The model under review builds one solid part; all positions refer to its coordinate system, in mm. A direction names the side the tool comes from. Round coordinates to 2 decimals unless told otherwise and drop trailing zeros. Write each loop counter-clockwise with the first axis right and the second up, starting at its lowest first coordinate (ties: lowest second). Pieces come first, ordered by that corner, then holes. Notation, with made-up numbers: M -23.75,18.5 L -10.75,18.5 A7 ccw -10.75,23.5 Z; hole C -16,47.25 d11. An arc over 180 degrees is marked long. One line per item, written item: value. Start each with the question number.
1) For P1, Ø1.5, axis at y = 19.5, z = 4, coming from the +X side; P2, Ø3.5, axis at x = -0.5, y = 53, coming from the -Z side; P3, Ø5, axis at x = 0.5, y = -52.5, coming from the -Z side (3 decimals); P4, Ø0.7, axis at x = 0.5, z = -2.5, coming from the -Y side, all flat-tipped, find the tip position at first contact; note any pin that passes through.
2) Take a section at A-A, the plane y = 11. Write out the cut boundary in (x, z) (1 decimal), and give its area (3 significant figures).
3) Tool access review of faces 1 (the face through (-2, 55.562, 2)), 2 (the face through (-0.69, 45.65, -3.1)), 3 (the face through (0, 53, 2.245)), 4 (the face through (2.245, -53, 0)): name each direction out of +Z, -Z, +X, -X, +Y, -Y from which nothing blocks a thin tool from reaching the whole face with its end or side.
4) Take a section at B-B, the plane y = 57. Write out the cut boundary in (x, z).
5) Wall thickness on probe 1 along Y at (x, z) = (3, -3.25); probe 2 along Z at (x, y) = (-1.5, 52); probe 3 along X at (y, z) = (57.5, -1.5): over which ranges is each line inside the solid? List them lowest first.
from build123d import *

# Parameters (mm, degrees)
F0_R     = 3.175
F1_DEPTH = 50.8
F2_W     = 4.490128
F2_H     = 4.490128
F3_DEPTH = 4.7625
F4_R     = 2.245064
F5_DEPTH = 12.7
F6_R     = 4.7625
F7_DEPTH = 40.64


with BuildPart() as f1:
    # F0 (on Front) → F1 (new body)
    with BuildSketch(Plane.XZ):
        Circle(F0_R)
    extrude(amount=F1_DEPTH)

    # F2 (on face) → F3 (join)
    with BuildSketch(Plane.XZ.offset(50.8)):
        Rectangle(F2_W, F2_H)
    extrude(amount=F3_DEPTH)

    # F4 (on face) → F5 (join)
    with BuildSketch(Plane.XZ.offset(55.5625)):
        Circle(F4_R)
    extrude(amount=F5_DEPTH)

    # F6 (on face) → F7 (join)
    with BuildSketch(Plane(origin=(0, 0, 0), x_dir=(-1, 0, 0), z_dir=(0, 1, 0))):
        Circle(F6_R)
    extrude(amount=-F7_DEPTH)

    # F8: F1 across plane


with BuildPart() as f1_1:
    add(f1.part)
    add(f1.part.mirror(Plane.XZ))


solid = f1_1.part
Checked values:
1. P1: stops at x = 3.48
1. P2: stops at z = -2.25
1. P3: stops at z = -3.175
1. P4: stops at y = -68.26
2. outline: C 0,0 d9.5
2. area: 71.3 mm2
3. face 1: +Z, -X, +Y
3. face 2: +Y
3. face 3: +Z, +X, -X, +Y
3. face 4: +Z, -Z, +X, -Y
4. outline: C 0,0 d4.49
5. probe 1: y = -40.64 to 40.64
5. probe 2: z = -2.25 to 2.25
5. probe 3: x = -1.67 to 1.67
